CAD build for the part. Positions are in the model's coordinates, mm. Face numbers are marked on the shaded views. A direction names the side the tool comes from. Give positions to 0.01 mm unless a question says otherwise; leave off trailing zeros. Order: outer loops, then holes, each group sorted by start corner. A loop starts at its lowest first (then second) coordinate and runs counter-clockwise, first axis right, second up. Notation, with made-up numbers: (84, 36) -> (103, 36) arc R30 cw to (103, 73) -> close; hole circle Ø11 at (15, 60). An arc over 180 degrees is marked (long way). Use one line per item in the form item = value. Start each with the question number.
1) Cut at D-D, the plane z = 13. State how many separate pieces and enclosed holes the cut face has, and give its area (3 significant figures).
2) Mould opens along Y. For the marked faces 1, 2 and 3 say: pulls with the +Y half, pulls with the -Y half, needs draft (parallel to the pull), parting line crosses it, or undercut.
3) Drop flat-ended pins along their axis: P1, Ø8, axis at x = 17, y = -26, coming from the +Z side (3 decimals); P2, Ø2, axis at x = 30.5, z = 19, coming from the -Y side; P3, Ø0.9, axis at x = 27, z = 0.5, coming from the -Y side. Give the stop position or say it passes through.
4) Tool access for the marked faces 4, 5, 6, 7 and 8: list every direction of +Z, -Z, +X, -X, +Y, -Y with a clear straight run to the whole face (end or side of a thin tool).
5) Cut at C-C, the plane y = -1.5. Give the cut face in (x, z), and give its area (3 significant figures).
6) Probe line 1 (X direction, y = -23, z = 23.5); line 2 (Y direction, x = 4.5, z = 23); line 3 (Y direction, x = 5.5, z = 16). List the from-to ranges inside material, lowest first.
7) Cut at B-B, the plane x = 18.5. Give the cut face in (y, z) (3 decimals), and give its area (3 significant figures).
8) Cut at A-A, the plane y = -24. Give the cut face in (x, z) (3 decimals).
from build123d import *

# Parameters (mm, degrees)
F0_W     = 38.1
F0_H     = 38.1
F1_DEPTH = 38.1
F3_DEPTH = 38.1
F5_DEPTH = 38.1
F7_W     = 7.62
F7_H     = 25.4
F7_H_2   = 30.48
F8_DEPTH = 38.1


with BuildPart() as f1:
    # F0 (on Front) → F1 (new body)
    with BuildSketch(Plane.XZ):
        with Locations((19.05, 19.05)):
            Rectangle(F0_W, F0_H)
    extrude(amount=F1_DEPTH)

    # F2 (on face) → F3 (cut)
    with BuildSketch(Plane.XZ.offset(38.1)):
        Polygon((31.75, 38.1), (6.35, 38.1), (11.43, 20.955), (16.51, 28.575), (21.59, 28.575), (26.67, 20.955), align=None)
        Polygon((0, 38.1), (0, 0), (6.35, 0), align=None)
        Polygon((19.05, 15.875), (19.05, 0), (25.4, 0), align=None)
        Polygon((19.05, 15.875), (12.7, 0), (19.05, 0), align=None)
        Polygon((38.1, 0), (38.1, 38.1), (31.75, 0), align=None)
    extrude(amount=-F3_DEPTH, mode=Mode.SUBTRACT)

    # F4 (on face) → F5 (cut)
    with BuildSketch(Plane(origin=(30.891892, 0, -5.148649), x_dir=(0, 1, 0), z_dir=(0.986394, 0, -0.164399))):
        Polygon((-6.35, 43.84521), (0, 5.219668), (0, 43.84521), align=None)
        Polygon((-12.7, 43.84521), (-19.05, 43.84521), (-19.05, 30.619668), align=None)
        Polygon((-19.05, 43.84521), (-25.4, 43.84521), (-19.05, 30.619668), align=None)
        Polygon((-26.67, 27.444668), (-31.75, 5.219668), (-6.35, 5.219668), (-11.43, 27.444668), (-16.51, 14.744668), (-21.59, 14.744668), align=None)
        Polygon((-31.75, 43.84521), (-38.1, 43.84521), (-38.1, 5.219668), align=None)
    extrude(amount=-F5_DEPTH, mode=Mode.SUBTRACT)

    # F7 (on offset) → F8 (cut)
    with BuildSketch(Plane.XY.offset(38.1)):
        with Locations((26.67, -25.4)):
            Rectangle(F7_W, F7_H)
        with Locations((11.43, -15.24)):
            Rectangle(F7_W, F7_H_2)
    extrude(amount=-F8_DEPTH, mode=Mode.SUBTRACT)


solid = f1.part
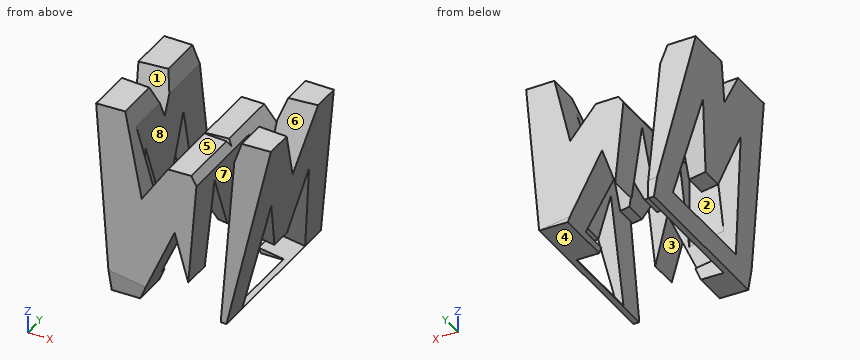
Result:
q1.separate_pieces = 9
q1.enclosed_holes = 0
q1.area = 331 mm²
q2.face_1 = undercut
q2.face_2 = pulls with the +Y half
q2.face_3 = needs draft
q3.P1 = 28.575
q3.P2 = -35.22
q3.P3 = -12.7
q4.face_4 = -Z, +X, -X, +Y, -Y
q4.face_5 = +Z, +Y, -Y
q4.face_6 = +Z, +X
q4.face_7 = +Z, -Z, -Y
q4.face_8 = +Z, -Z, +Y
q5.outline = (4.04, 13.87) -> (6.35, 0) -> (7.62, 0) -> (7.62, 13.27) -> close; (15.24, 6.35) -> (17.36, 11.65) -> (15.24, 12) -> close; (20.98, 11.04) -> (25.4, 0) -> (31.75, 0) -> (33.25, 9) -> close
q5.area = 130 mm²
q6.line_1 = 2.43 to 7.62, 15.24 to 22.86, 30.48 to 35.67
q6.line_2 = -35.11 to -27.59, -25.06 to -13.04, -10.51 to -2.99
q6.line_3 = -36.21 to -29.13, -22.37 to -15.73, -8.97 to -1.89
q7.outline = (-36.107, 14.5) -> (-28.979, 14.5) -> (-26.67, 24.74) -> (-22.63, 14.5) -> (-15.47, 14.5) -> (-11.43, 24.74) -> (-9.121, 14.5) -> (-1.993, 14.5) -> (-4.276, 28.575) -> (-18.758, 28.575) -> (-19.05, 27.959) -> (-19.342, 28.575) -> (-33.824, 28.575) -> close
q7.area = 383 mm²
q8.outline = (0, 38.1) -> (2.922, 20.569) -> (7.62, 19.786) -> (7.62, 33.814) -> (6.35, 38.1) -> close; (5.624, 4.354) -> (6.35, 0) -> (7.62, 0) -> (7.62, 4.022) -> close; (15.24, 18.516) -> (22.86, 17.246) -> (22.86, 26.67) -> (21.59, 28.575) -> (16.51, 28.575) -> (15.24, 26.67) -> close; (30.48, 0) -> (31.75, 0) -> (30.48, 0.212) -> close; (30.48, 15.976) -> (34.306, 15.338) -> (37.621, 35.224) -> (31.214, 36.292) -> (30.48, 33.814) -> close
